from build123d import *

# Parameters (mm, degrees)
F0_R          = 22.225
F0_R_2        = 17.315
F1_DEPTH      = 63.5
F4_SIZE       = 1
F5_R          = 4.9
F3_FACE_R     = 49.8
F3_FACE_R_2   = 22.225
F6_DEPTH      = 40
F7_DEPTH      = 63.501
F7_DEPTH_BACK = 30
F8_R          = 17.315
F9_DEPTH      = 12
F10_R         = 3
F11_R         = 33.5271440313
F12_DEPTH     = 7
F13_R         = 3
F14_W         = 5
F14_H         = 4.8698585015
F15_DEPTH     = 50.3537864045
F16_SIZE      = 1


# Not quite as in the source:
# - a feature names something its author has since deleted; it is built from what else it names


with BuildPart() as f1:
    # F0 (on Top) → F1 (new body)
    with BuildSketch(Plane.XY):
        Circle(F0_R)
        Circle(F0_R_2, mode=Mode.SUBTRACT)
    extrude(amount=F1_DEPTH)

    # F2 (on Right) → F3 (revolve)
    with BuildSketch(Plane.YZ):
        Polygon((-38.1, 0), (0, 0), (0, 25.4), (-17.315, 25.4), (-50.8, 25.4), align=None)
    revolve(axis=Axis((0, 0, 12.7), (0, 0, 1)))

    # F4
    f4_edges = [f1.edges().sort_by_distance(p)[0] for p in [
        (0, 50.8, 25.4),
    ]]
    chamfer(f4_edges, length=F4_SIZE)

    # F5 (on Top) + F3_face (on face) → F6 (cut)
    with BuildSketch(Plane.XY):
        Circle(F5_R)
    with BuildSketch(Plane.XY.offset(25.4)):
        Circle(F3_FACE_R)
        Circle(F3_FACE_R_2, mode=Mode.SUBTRACT)
    extrude(amount=F6_DEPTH, mode=Mode.SUBTRACT)

    # F5 (on Top) → F7 (cut, two sides)
    with BuildSketch(Plane.XY) as f7_sk:
        Circle(F5_R)
    extrude(amount=F7_DEPTH, mode=Mode.SUBTRACT)
    extrude(f7_sk.sketch, amount=-F7_DEPTH_BACK, mode=Mode.SUBTRACT)

    # F8 (on face) → F9 (cut)
    with BuildSketch(Plane.XY.offset(25.4)):
        Circle(F8_R)
    extrude(amount=-F9_DEPTH, mode=Mode.SUBTRACT)

    # F10
    f10_edges = [f1.edges().sort_by_distance(p)[0] for p in [
        (-17.315, 0, 13.4),
    ]]
    fillet(f10_edges, radius=F10_R)

    # F11 (on face) → F12 (cut)
    with BuildSketch(Plane(origin=(0, 0, 0), x_dir=(1, 0, 0), z_dir=(0, 0, -1))):
        Circle(F11_R)
    extrude(amount=-F12_DEPTH, mode=Mode.SUBTRACT)

    # F13
    f13_edges = [f1.edges().sort_by_distance(p)[0] for p in [
        (-33.527144, 0, 7),
    ]]
    fillet(f13_edges, radius=F13_R)

    # F14 (on Right) → F15 (cut, through all)
    with BuildSketch(Plane.YZ):
        with BuildLine():
            Line((-2.4888959483, 2.3854229395), (-2.5063311768, 0))
            Line((-2.5063311768, 0), (2.4936688232, 0))
            Line((2.4936688232, 0), (2.4921056953, 2.4222710093))
            ThreePointArc((2.4921056953, 2.4222710093), (0.0184938011, 0.120856929), (-2.4888959483, 2.3854229395))
        make_face()
        with Locations((-0.0063311768, -2.4349292507)):
            Rectangle(F14_W, F14_H)
        with BuildLine():
            Line((-2.485189612, 2.8925100588), (-2.4888959483, 2.3854229395))
            ThreePointArc((-2.4888959483, 2.3854229395), (0.0184938011, 0.120856929), (2.4921056953, 2.4222710093))
            Line((2.4921056953, 2.4222710093), (2.4918474071, 2.8225222584))
            ThreePointArc((2.4918474071, 2.8225222584), (0.0351518792, 5.1205413808), (-2.485189612, 2.8925100588))
        make_face()
        with BuildLine():
            ThreePointArc((-2.485189612, 2.8925100588), (-2.4999332245, 2.6390607164), (-2.4888959483, 2.3854229395))
            Line((-2.4888959483, 2.3854229395), (-2.485189612, 2.8925100588))
        make_face()
        with BuildLine():
            Line((2.4918474071, 2.8225222584), (2.4921056953, 2.4222710093))
            ThreePointArc((2.4921056953, 2.4222710093), (2.4980256442, 2.5214513158), (2.5, 2.6207885239))
            ThreePointArc((2.5, 2.6207885239), (2.4979610203, 2.7217377245), (2.4918474071, 2.8225222584))
        make_face()
    extrude(amount=-F15_DEPTH, mode=Mode.SUBTRACT)

    # F16
    f16_edges = [f1.edges().sort_by_distance(p)[0] for p in [
        (-22.225, 0, 25.4),
    ]]
    chamfer(f16_edges, length=F16_SIZE)


solid = f1.part
Verification items for the finished model (mm, model axes). A direction names the side the tool comes from. Coordinates: 2 decimals unless noted, no trailing zeros. Write each loop counter-clockwise with the first axis right and the second up, starting at its lowest first coordinate (ties: lowest second). Pieces come first, ordered by that corner, then holes. Notation, with made-up numbers: (54, -10.75) -> (84, -10.75) arc R21 cw to (84, 0.25) -> close; hole circle Ø6 at (32.25, 31). An arc over 180 degrees is marked (long way). One line per item, written item: value. Start each with the question number.
Q1. Cross-section at C-C on z = 58. Enter the section's corners in (x, y) (3 decimals), and give its area (3 significant figures).
Q2. Access from +Z, -Z, +X, -X, +Y, -Y to the whole of each face (thin tool, end or side, straight path). Record for faces 5 (the cylindrical face through (-1.062, -4.783, 10.155)), 6 (the cylindrical face through (-13.741, -10.536, 40.28)), 7 (the cylindrical face through (33.496, 1.445, 1.972)).
Q3. Thickness scan on L1, parallel to Y at x = 0, z = 30 (3 decimals); L2, parallel to Z at x = 5, y = 20.5; L3, parallel to X at y = 7, z = 30. Record the ranges inside material, lowest first. Write a range as from..to.
Q4. Mould release check, pull along X, two halves, no side actions. Record for faces 1 (the conical face through (-37.775, 8.388, 1.19)), 2 (the flat face through (0, 6, 7)), 3 (the flat face through (6, 0, 13.4)), 4 (the flat face through (-10.4, 21.4, 25.4)): pulls with the +X half, pulls with the -X half, needs draft (parallel to the pull), parting line crosses it, or undercut.
Q5. Cross-section at A-A on x = 0. Enter the section's corners in (y, z) (3 decimals), and give its area (3 significant figures).
Q6. Cross-section at B-B on y = 0. Enter the section's corners in (x, z) (3 decimals), and give its area (3 significant figures).
Q7. Go/stop test with flat-tipped pins: P1, Ø5, axis at x = 23, z = 44, coming from the -Y side; P2, Ø10, axis at x = -34.5, y = -21, coming from the -Z side; P3, Ø3, axis at x = 18, y = -37.5, coming from the +Z side; P4, Ø2, axis at x = 37.5, z = 21.5, coming from the -Y side. Record where each tip stops, or that it passes through.
Checked values:
1. outline: circle Ø44.45 at (0, 0); hole circle Ø34.63 at (0, 0)
1. area: 610 mm²
2. face 5: +Z, -Z
2. face 6: +Z
2. face 7: -Z
3. L1: y = -22.225..-17.315, 17.315..22.225
3. L2: z = 7..63.5
3. L3: x = -21.09..-15.84, 15.84..21.09
4. face 1: parting line crosses it
4. face 2: undercut
4. face 3: undercut
4. face 4: needs draft
5. outline: (-50.353, 24.506) -> (-38.1, 0) -> (-33.527, 0) -> (-33.527, 4) arc R3 cw to (-30.527, 7) -> (-4.9, 7) -> (-4.9, 13.4) -> (-14.315, 13.4) arc R3 cw to (-17.315, 16.4) -> (-17.315, 63.5) -> (-22.225, 63.5) -> (-22.225, 26.4) -> (-23.225, 25.4) -> (-49.8, 25.4) -> close; (4.9, 7) -> (30.527, 7) arc R3 cw to (33.527, 4) -> (33.527, 0) -> (38.1, 0) -> (50.353, 24.506) -> (49.8, 25.4) -> (23.225, 25.4) -> (22.225, 26.4) -> (22.225, 63.5) -> (17.315, 63.5) -> (17.315, 16.4) arc R3 cw to (14.315, 13.4) -> (4.9, 13.4) -> close
5. area: 1,690 mm²
6. outline: (-50.353, 24.506) -> (-40.66, 5.121) -> (-33.31, 5.121) arc R3 cw to (-30.527, 7) -> (-4.9, 7) -> (-4.9, 13.4) -> (-14.315, 13.4) arc R3 cw to (-17.315, 16.4) -> (-17.315, 63.5) -> (-22.225, 63.5) -> (-22.225, 26.4) -> (-23.225, 25.4) -> (-49.8, 25.4) -> close; (4.9, 7) -> (30.527, 7) arc R3 cw to (33.527, 4) -> (33.527, 0) -> (38.1, 0) -> (50.353, 24.506) -> (49.8, 25.4) -> (23.225, 25.4) -> (22.225, 26.4) -> (22.225, 63.5) -> (17.315, 63.5) -> (17.315, 16.4) arc R3 cw to (14.315, 13.4) -> (4.9, 13.4) -> close
6. area: 1,660 mm²
7. P1: stops at y = -8.58
7. P2: stops at z = 0
7. P3: stops at z = 25.4
7. P4: stops at y = -32.69
